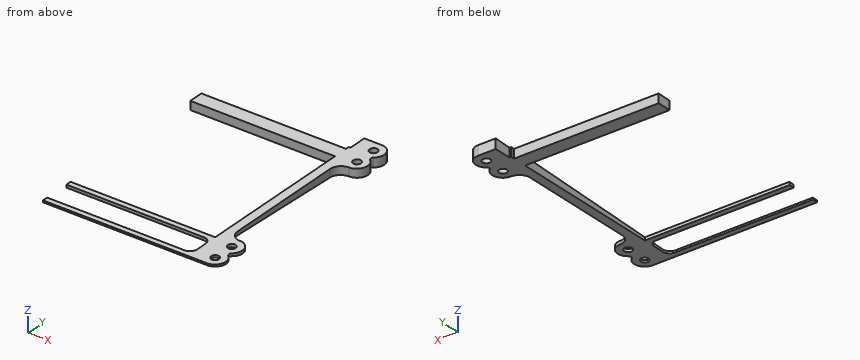
```python
from build123d import *

# Parameters (mm, degrees)
BOSS_EXTRUDE1_OUTLINE_R = 3.556
BOSS_EXTRUDE1_OUTLINE_W = 260.9469
BOSS_EXTRUDE1_OUTLINE_H = 138.1252
BOSS_EXTRUDE1_DEPTH     = 76.2
CUT_EXTRUDE1_DEPTH      = 355.32482824
CUT_EXTRUDE1_DEPTH_BACK = 355.32482824
FILLET1_R               = 2.54
SKETCH7_W               = 260.9469
SKETCH7_H               = 22.1996
CUT_EXTRUDE2_DEPTH      = 347.152897849
FILLET2_R               = 6.35
SKETCH8_W               = 208.809057266
SKETCH8_H               = 235.521960295
CUT_EXTRUDE4_DEPTH      = 347.144751077


# Read off the part's stored shape, not the designer's step: Boss-Extrude1
with BuildPart() as part:
    # Boss-Extrude1 outline → Boss-Extrude1 (new body)
    with BuildSketch(Plane.XY):
        with BuildLine():
            Line((-286.3596, -22.225), (9.525, -22.225))
            ThreePointArc((9.525, -22.225), (19.05, -12.7), (9.525, -3.175))
            ThreePointArc((9.525, -3.175), (19.05, 6.35), (9.525, 15.875))
            ThreePointArc((9.525, 15.875), (2.789807909, 18.664807909), (0, 25.4))
            Line((0, 25.4), (0, 131.7752))
            ThreePointArc((0, 131.7752), (2.789807909, 138.510392091), (9.525, 141.3002))
            ThreePointArc((9.525, 141.3002), (19.05, 150.8252), (9.525, 160.3502))
            ThreePointArc((9.525, 160.3502), (19.05, 169.8752), (9.525, 179.4002))
            Line((9.525, 179.4002), (-6.35, 179.4002))
            Line((-6.35, 179.4002), (-6.35, 163.5252))
            Line((-6.35, 163.5252), (-7.9502, 163.5252))
            Line((-7.9502, 163.5252), (-7.9502, 160.3502))
            Line((-7.9502, 160.3502), (-268.9098, 160.3502))
            Line((-268.9098, 160.3502), (-268.9098, 163.5252))
            Line((-268.9098, 163.5252), (-270.51, 163.5252))
            Line((-270.51, 163.5252), (-270.51, 179.4002))
            Line((-270.51, 179.4002), (-286.385, 179.4002))
            ThreePointArc((-286.385, 179.4002), (-295.91, 169.8752), (-286.385, 160.3502))
            ThreePointArc((-286.385, 160.3502), (-295.897297883, 150.818850004), (-286.3723, 141.3002))
            ThreePointArc((-286.3723, 141.3002), (-279.637107909, 138.510392091), (-276.8473, 131.7752))
            Line((-276.8473, 131.7752), (-276.8473, 25.4))
            ThreePointArc((-276.8473, 25.4), (-279.637107909, 18.664807909), (-286.3723, 15.875))
            ThreePointArc((-286.3723, 15.875), (-295.8973, 6.35), (-286.3723, -3.175))
            ThreePointArc((-286.3723, -3.175), (-295.884597883, -12.706349996), (-286.3596, -22.225))
        make_face()
        with Locations((-286.3596, -12.7)):
            Circle(BOSS_EXTRUDE1_OUTLINE_R, mode=Mode.SUBTRACT)
        with Locations((-286.3723, 6.35)):
            Circle(BOSS_EXTRUDE1_OUTLINE_R, mode=Mode.SUBTRACT)
        with Locations((9.525, -12.7)):
            Circle(BOSS_EXTRUDE1_OUTLINE_R, mode=Mode.SUBTRACT)
        with Locations((9.525, 6.35)):
            Circle(BOSS_EXTRUDE1_OUTLINE_R, mode=Mode.SUBTRACT)
        with Locations((-286.3723, 150.8252)):
            Circle(BOSS_EXTRUDE1_OUTLINE_R, mode=Mode.SUBTRACT)
        with Locations((-286.385, 169.8752)):
            Circle(BOSS_EXTRUDE1_OUTLINE_R, mode=Mode.SUBTRACT)
        with Locations((-138.42365, 78.5876)):
            Rectangle(BOSS_EXTRUDE1_OUTLINE_W, BOSS_EXTRUDE1_OUTLINE_H, mode=Mode.SUBTRACT)
        with Locations((9.525, 150.8252)):
            Circle(BOSS_EXTRUDE1_OUTLINE_R, mode=Mode.SUBTRACT)
        with Locations((9.525, 169.8752)):
            Circle(BOSS_EXTRUDE1_OUTLINE_R, mode=Mode.SUBTRACT)
    extrude(amount=BOSS_EXTRUDE1_DEPTH)

    # Sketch5 → Cut-Extrude1 (cut, two sides: drawn at the far end of the back side and taken through both)
    with BuildSketch(Plane.ZY.offset(276.8473).offset(-CUT_EXTRUDE1_DEPTH_BACK)):
        Polygon((1.6002, -22.225), (8.641107133, 179.4002), (76.2, 179.4002), (76.2, -22.225), align=None)
    extrude(amount=CUT_EXTRUDE1_DEPTH + CUT_EXTRUDE1_DEPTH_BACK, mode=Mode.SUBTRACT)

    # Fillet1
    fillet1_edges = [part.edges().sort_by_distance(p)[0] for p in [
        (-286.385, 160.3502, 3.987933237),
        (-286.3723, -3.175, 1.132720329),
        (9.525, -3.175, 1.132720329),
        (9.525, 160.3502, 3.987933237),
    ]]
    fillet(fillet1_edges, radius=FILLET1_R)

    # Sketch7 → Cut-Extrude2 (cut, through all)
    with BuildSketch(Plane(origin=(0, 0, 0), x_dir=(-1, 0, 0), z_dir=(0, 0, -1))):
        with Locations((138.42365, -6.35)):
            Rectangle(SKETCH7_W, SKETCH7_H)
    extrude(amount=-CUT_EXTRUDE2_DEPTH, mode=Mode.SUBTRACT)

    # Fillet2
    fillet2_edges = [part.edges().sort_by_distance(p)[0] for p in [
        (-268.8971, 4.7498, 1.271090386),
        (-268.8971, -17.4498, 0.883476829),
        (-7.9502, -17.4498, 0.883476829),
        (-7.9502, 4.7498, 1.271090386),
    ]]
    fillet(fillet2_edges, radius=FILLET2_R)

    # Sketch8 → Cut-Extrude4 (cut, through all)
    with BuildSketch(Plane(origin=(0, -0.082881646, 2.373419811), x_dir=(1, 0, 0), z_dir=(0, -0.03489949670250444, 0.9993908270190958))):
        with Locations((-242.828178633, 74.917246318)):
            Rectangle(SKETCH8_W, SKETCH8_H)
    extrude(amount=-CUT_EXTRUDE4_DEPTH, mode=Mode.SUBTRACT)


solid = part.part
```
The model under review builds one solid part; all positions refer to its coordinate system, in mm. Coordinates: 2 decimals unless noted, no trailing zeros. Order: outer loops, then holes, each group sorted by start corner. A loop starts at its lowest first (then second) coordinate and runs counter-clockwise, first axis right, second up. Notation, with made-up numbers: (35, 3) -> (70, 3) arc R15 ccw to (70, 15) -> close; hole circle Ø7 at (-21.5, 82.5). An arc over 180 degrees is marked (long way). Answer in a Markdown table with one row per item. Add a question column.
Item 1: Clearance check with flat-ended pins moving along their axes: pin 1 (1.2 mm diameter, centred on y = -5.5, z = 0.5, fed in from -X); pin 2 (3 mm diameter, centred on x = -48, z = 1, fed in from +Y); pin 3 (8 mm diameter, centred on x = 9.52, y = 150.83, fed in from +Z). State where each tip first meets the part, or that it passes through.
Item 2: We need section C-C on z = 5.25. Give the number of separate pieces and of enclosed holes in the cut face, plus the area to 3 significant figures.
Item 3: We need section A-A on x = -93. Write out the cut boundary in (y, z) (3 decimals).
Item 4: We need section B-B on y = 75.5. Write out the cut boundary in (x, z).
Item 5: To check wall thickness, follow probe 1 along Y at (x, z) = (-24.5, 1) (3 decimals); probe 2 along X at (y, z) = (6.35, 1.8); probe 3 along Y at (x, z) = (-26.5, 5). State the ranges of each line that lie inside material, in increasing order.
Final values:
| question | item | result |
|---|---|---|
| 1 | pin 1 | stops at x = -7.95 |
| 1 | pin 2 | stops at y = 160.35 |
| 1 | pin 3 | stops at z = 7.78 |
| 2 | separate pieces | 1 |
| 2 | enclosed holes | 2 |
| 2 | area | 3,000 mm2 |
| 3 | outline | (-22.225, 0) -> (-17.45, 0) -> (-17.45, 1.767) -> (-22.225, 1.6) -> close; (4.75, 0) -> (9.525, 0) -> (9.525, 2.709) -> (4.75, 2.542) -> close; (147.65, 0) -> (160.35, 0) -> (160.35, 7.976) -> (147.65, 7.532) -> close |
| 4 | outline | (-7.95, 0) -> (0, 0) -> (0, 5.01) -> (-7.95, 5.01) -> close |
| 5 | probe 1 | y = -22.225 to -17.45, 4.75 to 9.525, 147.65 to 160.35 |
| 5 | probe 2 | x = -138.42 to 5.97, 13.08 to 19.05 |
| 5 | probe 3 | y = 147.65 to 160.35 |
